Build history of the part. All positions in model axes, mm. Give positions to 0.01 mm unless a question says otherwise; leave off trailing zeros. Order: outer loops, then holes, each group sorted by start corner. A loop starts at its lowest first (then second) coordinate and runs counter-clockwise, first axis right, second up. Notation, with made-up numbers: (43, -33) -> (75, -33) arc R31 ccw to (75, -9) -> close; hole circle Ø2 at (40, -14.5). An arc over 180 degrees is marked (long way). Write item = value, one per line. Start each with the question number.
from build123d import *

# Parameters (mm, degrees)
SKETCH_1_W               = 150
SKETCH_1_H               = 92
SKETCH_1_R               = 35
EXTRUDE_1_DEPTH          = 3
CUT_EXTRUDE_1_REACH      = 90.034
SKETCH_2_R               = 2
PATTERN_CIRCULAR_1_COUNT = 10
SKETCH_3_R               = 1.5
CUT_EXTRUDE_2_DEPTH      = 3
FILLET_1_R               = 10


with BuildPart() as part:
    # 草圖1 → 填料-伸長1 (new body)
    with BuildSketch(Plane(origin=(0, 0, 0), x_dir=(1, 0, 0), z_dir=(0, 1, 0))):
        Rectangle(SKETCH_1_W, SKETCH_1_H)
        with Locations(Location((15, 0, 0), (0, 0, 270))):
            Circle(SKETCH_1_R, mode=Mode.SUBTRACT)
    extrude(amount=EXTRUDE_1_DEPTH)

    # 草圖2 → 除料-伸長1 (cut, up to next)
    with BuildSketch(Plane(origin=(0, 3, 0), x_dir=(1, 0, 0), z_dir=(0, 1, 0)), mode=Mode.PRIVATE) as cut_extrude_1_sk1:
        with Locations(Location((57, 0, 0), (0, 0, 270))):
            Circle(SKETCH_2_R)
    cut_extrude_1_tool1 = extrude(cut_extrude_1_sk1.sketch, amount=-CUT_EXTRUDE_1_REACH, mode=Mode.PRIVATE) & part.part
    cut_extrude_1 = cut_extrude_1_tool1.solids().sort_by_distance((57, 3, 0))[0]
    add(cut_extrude_1, mode=Mode.SUBTRACT)

    # 環狀複製排列1: 除料-伸長1 ×10 about axis
    pattern_circular_1_axis = Axis((15, 0, 0), (0, 1, 0))
    for i in range(1, PATTERN_CIRCULAR_1_COUNT):
        add(cut_extrude_1.rotate(pattern_circular_1_axis, i * 360 / PATTERN_CIRCULAR_1_COUNT), mode=Mode.SUBTRACT)

    # 草圖3 → 除料-伸長2 (cut)
    with BuildSketch(Plane(origin=(0, 3, 0), x_dir=(1, 0, 0), z_dir=(0, 1, 0))):
        with Locations(Location((-67, 32, 0), (0, 0, 270))):
            Circle(SKETCH_3_R)
        with Locations(Location((-67, 18, 0), (0, 0, 270))):
            Circle(SKETCH_3_R)
        with Locations(Location((-43, 18, 0), (0, 0, 90))):
            Circle(SKETCH_3_R)
        with Locations(Location((-43, 32, 0), (0, 0, 90))):
            Circle(SKETCH_3_R)
        with Locations(Location((-55, -10, 0), (0, 0, 270))):
            Circle(SKETCH_3_R)
        with Locations(Location((-55, -30, 0), (0, 0, 270))):
            Circle(SKETCH_3_R)
    extrude(amount=-CUT_EXTRUDE_2_DEPTH, mode=Mode.SUBTRACT)

    # 圓角1
    fillet_1_edges = [part.edges().sort_by_distance(p)[0] for p in [
        (75, 1.5, 46),
        (-75, 1.5, 46),
        (-75, 1.5, -46),
        (75, 1.5, -46),
    ]]
    fillet(fillet_1_edges, radius=FILLET_1_R)


solid = part.part
(1) Mould opens along X. For faces 1 (the face through (-20.43, 1.521, 26.063)), 2 (the face through (-18, 3, -21)), 3 (the face through (-75, 1, 1)), 4 (the face through (28.34, 1.52, -41.91)) say: released by +X, released by -X, zero draft, split by the parting line, or undercut.
(2) Cut at A-A, the plane x = 15. Give the cut face in (y, z), plus the area to 3 significant figures.
(3) Cut at D-D, the plane z = 30. Give the cut face in (x, y).
(4) Cut at B-B, the plane z = 0. Give the cut face in (x, y).
(5) Cut at C-C, the plane x = -55. Give the cut face in (y, z).
(6) Wall check: line 1 (Z direction, x = -43, y = 1.4); line 2 (X direction, y = 0.9, z = -18); line 3 (Z direction, x = -56, y = 0.4). Give the ranges that are in metal, low to high. Write a range as [from, to].
Results:
q1.face_1 = undercut
q1.face_2 = zero draft
q1.face_3 = released by -X
q1.face_4 = undercut
q2.outline = (0, -46) -> (3, -46) -> (3, -35) -> (0, -35) -> close; (0, 35) -> (3, 35) -> (3, 46) -> (0, 46) -> close
q2.area = 66.0 mm2
q3.outline = (-75, 0) -> (-56.5, 0) -> (-56.5, 3) -> (-75, 3) -> close; (-53.5, 0) -> (-3.03, 0) -> (-3.03, 3) -> (-53.5, 3) -> close; (33.03, 0) -> (75, 0) -> (75, 3) -> (33.03, 3) -> close
q4.outline = (-75, 0) -> (-29, 0) -> (-29, 3) -> (-75, 3) -> close; (-25, 0) -> (-20, 0) -> (-20, 3) -> (-25, 3) -> close; (50, 0) -> (55, 0) -> (55, 3) -> (50, 3) -> close; (59, 0) -> (75, 0) -> (75, 3) -> (59, 3) -> close
q5.outline = (0, -46) -> (3, -46) -> (3, 8.5) -> (0, 8.5) -> close; (0, 11.5) -> (3, 11.5) -> (3, 28.5) -> (0, 28.5) -> close; (0, 31.5) -> (3, 31.5) -> (3, 46) -> (0, 46) -> close
q6.line_1 = [-46, -33.5], [-30.5, -19.5], [-16.5, 46]
q6.line_2 = [-75, -68.5], [-65.5, -44.5], [-41.5, -15.02], [45.02, 75]
q6.line_3 = [-46, 8.88], [11.12, 28.88], [31.12, 46]
